Verification items for the finished model (mm, model axes). Face numbers are marked on the shaded views. A direction names the side the tool comes from. Coordinates: 2 decimals unless noted, no trailing zeros. Order: outer loops, then holes, each group sorted by start corner. A loop starts at its lowest first (then second) coordinate and runs counter-clockwise, first axis right, second up. Notation, with made-up numbers: (56, 34) - (111, 34) arc R31 ccw to (111, 59) - close; hole circle Ø3 at (43, -21.75). An arc over 180 degrees is marked (long way). Answer as CSV lines item,"result". Start each with the question number.
1. Set-up check for the marked faces 1, 2, 3 and 4: record each of +Z, -Z, +X, -X, +Y, -Y from which the full face is reachable in a straight line by a thin tool's end or side.
2. Section check C-C (z = -9.5). Record the cut outline in (x, y), and give its area (3 significant figures).
3. Material ranges on L1, parallel to X at y = -112.25, z = 10; L2, parallel to Y at x = 10, z = 9; L3, parallel to Y at x = 15.85, z = 10.5, recorded low to high. Write a range as [from, to].
4. Section check B-B (x = 37.5). Record the cut outline in (y, z).
5. Mould release check, pull along Y, two halves, no side actions. Record for the marked faces 5, 6, 7 and 8: pulls with the +Y half, pulls with the -Y half, needs draft (parallel to the pull), parting line crosses it, or undercut.
6. Go/stop test with flat-tipped pins: pin 1 (11 mm diameter, centred on x = 10, y = -10, fed in from -Z); pin 2 (6 mm diameter, centred on x = 26, z = -2.5, fed in from +Y); pin 3 (7.5 mm diameter, centred on y = -62, z = 3.5, fed in from +X). Record where each tip stops, or that it passes through.
7. Section check A-A (y = -10). Record the cut outline in (x, z), and give its area (3 significant figures).
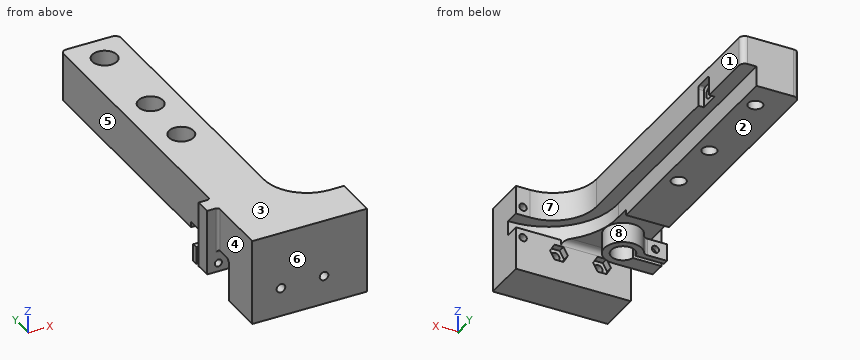
from build123d import *

# Parameters (mm, degrees)
BOSS_EXTRUDE1_DEPTH = 17
SKETCH3_W           = 40
SKETCH3_H           = 15
BOSS_EXTRUDE3_DEPTH = 13
FILLET1_R           = 15
SKETCH4_R           = 1.5000000000000004
SKETCH4_R_2         = 1.5000000000000007
CUT_EXTRUDE1_DEPTH  = 20
CUT_EXTRUDE2_DEPTH  = 2.5
SKETCH6_R           = 4.299999999999999
SKETCH6_R_2         = 4.299999999999998
SKETCH6_R_3         = 4.3
CUT_EXTRUDE3_DEPTH  = 12
SKETCH7_R           = 2.5000000000000004
SKETCH7_R_2         = 2.500000000000001
CUT_EXTRUDE4_DEPTH  = 12
CUT_EXTRUDE5_DEPTH  = 2
BOSS_EXTRUDE4_DEPTH = 23
BOSS_EXTRUDE5_DEPTH = 6
SKETCH11_W          = 6
SKETCH11_H          = 2
BOSS_EXTRUDE6_DEPTH = 4.419259302
SKETCH12_R          = 1.2500000000000002
CUT_EXTRUDE7_DEPTH  = 10
FILLET4_R           = 0.95
FILLET6_R           = 2
SKETCH13_R          = 6.500000000000007
SKETCH13_R_2        = 2.150000000000001
BOSS_EXTRUDE7_DEPTH = 1
SKETCH14_W          = 13.249650970727469
SKETCH14_H          = 1.5
CUT_EXTRUDE8_DEPTH  = 7
BOSS_EXTRUDE8_DEPTH = 10
SKETCH16_R          = 4.100000000000001
CUT_EXTRUDE9_DEPTH  = 6
CUT_EXTRUDE10_DEPTH = 5
SKETCH18_R          = 24.032057078793116
CUT_EXTRUDE11_DEPTH = 5
SKETCH20_R          = 1.3000000000000016
CUT_EXTRUDE12_DEPTH = 10
FILLET7_R           = 0.5
FILLET8_R           = 2
FILLET9_R           = 2
FILLET10_R          = 1
FILLET11_R          = 1
CUT_EXTRUDE15_DEPTH = 2
SKETCH24_R          = 2
CUT_EXTRUDE16_DEPTH = 5


with BuildPart() as part:
    # Sketch1 → Boss-Extrude1 (new body)
    with BuildSketch(Plane.XY):
        Polygon((0, 0), (1.531e-14, -125), (40.000000000000014, -125), (40.000000000000014, -110), (20.000000000000014, -110), (20.000000000000014, 0), align=None)
    extrude(amount=BOSS_EXTRUDE1_DEPTH)

    # Sketch3 → Boss-Extrude3 (add)
    with BuildSketch(Plane(origin=(0, 0, 0), x_dir=(-1, 0, 0), z_dir=(0, 0, -1))):
        with Locations((-20.000000000000014, -117.50000000000001)):
            Rectangle(SKETCH3_W, SKETCH3_H)
    extrude(amount=BOSS_EXTRUDE3_DEPTH)

    # Fillet1
    fillet1_edges = [part.edges().sort_by_distance(p)[0] for p in [
        (20.000000000000014, -110, 8.5),
    ]]
    fillet(fillet1_edges, radius=FILLET1_R)

    # Sketch4 → Cut-Extrude1 (cut)
    with BuildSketch(Plane.XZ.offset(125)):
        with Locations(Location((10.000000000000016, -2.999999999999999, 0), (0, 0, 270))):
            Circle(SKETCH4_R)
        with Locations(Location((25.000000000000014, -2.999999999999999, 0), (0, 0, 270))):
            Circle(SKETCH4_R_2)
    extrude(amount=-CUT_EXTRUDE1_DEPTH, mode=Mode.SUBTRACT)

    # Sketch5 → Cut-Extrude2 (cut)
    with BuildSketch(Plane(origin=(0, -110, 0), x_dir=(1, 0, 0), z_dir=(0, 1, 0))):
        Polygon((6.882308546376037, 3.0000000000000013), (8.441154273188026, 0.2999999999999986), (11.558845726812006, 0.2999999999999995), (13.117691453623996, 3.0000000000000018), (11.558845726812008, 5.7), (8.441154273188026, 5.699999999999998), align=None)
        Polygon((21.882308546376034, 2.999999999999999), (23.441154273188026, 0.2999999999999969), (26.558845726812, 0.29999999999999777), (28.117691453623994, 2.999999999999999), (26.558845726812, 5.6999999999999975), (23.441154273188022, 5.699999999999997), align=None)
    extrude(amount=-CUT_EXTRUDE2_DEPTH, mode=Mode.SUBTRACT)

    # Sketch6 → Cut-Extrude3 (cut)
    with BuildSketch(Plane.XY.offset(17)):
        with Locations((10.000000000000009, -10.000000000000002)):
            Circle(SKETCH6_R)
        with Locations((10.000000000000012, -40)):
            Circle(SKETCH6_R_2)
        with Locations((10.000000000000014, -60)):
            Circle(SKETCH6_R_3)
    extrude(amount=-CUT_EXTRUDE3_DEPTH, mode=Mode.SUBTRACT)

    # Sketch7 → Cut-Extrude4 (cut)
    with BuildSketch(Plane.XY.offset(5.000000000000001)):
        with Locations((10.000000000000009, -10.000000000000002)):
            Circle(SKETCH7_R)
        with Locations((10.000000000000012, -40)):
            Circle(SKETCH7_R_2)
        with Locations((10.000000000000014, -60)):
            Circle(SKETCH7_R_2)
    extrude(amount=-CUT_EXTRUDE4_DEPTH, mode=Mode.SUBTRACT)

    # Sketch8 → Cut-Extrude5 (cut)
    with BuildSketch(Plane(origin=(0, 0, 0), x_dir=(-1, 0, 0), z_dir=(0, 0, -1))):
        Polygon((-1.531e-14, -110), (-3.06e-15, -84.99999999999999), (-40.000000000000014, -84.99999999999999), (-40.000000000000014, -110), align=None)
    extrude(amount=-CUT_EXTRUDE5_DEPTH, mode=Mode.SUBTRACT)

    # Sketch9 → Boss-Extrude4 (add)
    with BuildSketch(Plane.XY.offset(17)):
        Polygon((-2.69e-15, -103.00000000000001), (-4, -103.00000000000001), (-4, -97.5), (0, -97.5), align=None)
    extrude(amount=-BOSS_EXTRUDE4_DEPTH)

    # Sketch10 → Boss-Extrude5 (add)
    with BuildSketch(Plane(origin=(0, 0, -5.999999999999998), x_dir=(-1, 0, 0), z_dir=(0, 0, -1))):
        with BuildLine():
            Line((4, -103.00000000000001), (-9.9, -103.00000000000001))
            ThreePointArc((-9.9, -103.00000000000001), (-15.308326913195994, -92.894448724536), (-3.8999999999999964, -94))
            Line((-3.8999999999999964, -94), (-0.41925930159213404, -94))
            Line((-0.41925930159213404, -94), (-0.41925930159213404, -96))
            Line((-0.41925930159213404, -96), (-5.931373033403113, -96))
            ThreePointArc((-5.931373033403113, -96), (-13.892119004323362, -96.24903017049799), (-6.025237793012059, -97.49308501111332))
            Line((-6.025237793012059, -97.49308501111332), (4, -97.5))
            Line((4, -97.5), (4, -103.00000000000001))
        make_face()
    extrude(amount=-BOSS_EXTRUDE5_DEPTH)

    # Sketch11 → Boss-Extrude6 (add)
    with BuildSketch(Plane.ZY.offset(-0.41925930159213404)):
        with Locations((-2.9999999999999982, -95)):
            Rectangle(SKETCH11_W, SKETCH11_H)
    extrude(amount=BOSS_EXTRUDE6_DEPTH)

    # Sketch12 → Cut-Extrude7 (cut)
    with BuildSketch(Plane(origin=(0, -94, 0), x_dir=(1, 0, 0), z_dir=(0, 1, 0))):
        with Locations((-0.05000000000000317, 2.9999999999999982)):
            Circle(SKETCH12_R)
    extrude(amount=-CUT_EXTRUDE7_DEPTH, mode=Mode.SUBTRACT)

    # Fillet4
    fillet4_edges = [part.edges().sort_by_distance(p)[0] for p in [
        (0, -97.5, 9.5),
        (-2.69e-15, -103.00000000000001, 9.5),
    ]]
    fillet(fillet4_edges, radius=FILLET4_R)

    # Fillet6
    fillet6_edges = [part.edges().sort_by_distance(p)[0] for p in [
        (20.000000000000014, 0, 8.5),
        (0, 0, 8.5),
    ]]
    fillet(fillet6_edges, radius=FILLET6_R)

    # Sketch13 → Boss-Extrude7 (add)
    with BuildSketch(Plane.XY):
        with Locations(Location((9.9, -96.5, 0), (0, 0, 175.588274214))):
            Circle(SKETCH13_R)
        with Locations((9.9, -96.5)):
            Circle(SKETCH13_R_2, mode=Mode.SUBTRACT)
    extrude(amount=BOSS_EXTRUDE7_DEPTH)

    # Sketch14 → Cut-Extrude8 (cut)
    with BuildSketch(Plane(origin=(0, 0, -5.999999999999998), x_dir=(-1, 0, 0), z_dir=(0, 0, -1))):
        with Locations((-2.6248254853637345, -96.75)):
            Rectangle(SKETCH14_W, SKETCH14_H)
    extrude(amount=-CUT_EXTRUDE8_DEPTH, mode=Mode.SUBTRACT)

    # Sketch15 → Boss-Extrude8 (add)
    with BuildSketch(Plane.XY):
        Polygon((0, -97.5), (2.5, -97.5), (2.5000000000000013, -103.00000000000001), (0, -103.00000000000001), align=None)
    extrude(amount=BOSS_EXTRUDE8_DEPTH)

    # Sketch16 → Cut-Extrude9 (cut)
    with BuildSketch(Plane(origin=(0, 0, -5.999999999999998), x_dir=(-1, 0, 0), z_dir=(0, 0, -1))):
        with Locations((-9.9, -96.5)):
            Circle(SKETCH16_R)
    extrude(amount=-CUT_EXTRUDE9_DEPTH, mode=Mode.SUBTRACT)

    # Sketch17 → Cut-Extrude10 (cut)
    with BuildSketch(Plane(origin=(20.000000000000014, 0, 0), x_dir=(0, 0, -1), z_dir=(1, 0, 0))):
        Polygon((0, 0), (-7, -8.6e-16), (-6.9999999999999885, -89.75912634068962), (0, -89.75912634068962), align=None)
    extrude(amount=-CUT_EXTRUDE10_DEPTH, mode=Mode.SUBTRACT)

    # Sketch18 → Cut-Extrude11 (cut)
    with BuildSketch(Plane(origin=(0, 0, 2), x_dir=(-1, 0, 0), z_dir=(0, 0, -1))):
        with Locations((-39.000000000000014, -91)):
            Circle(SKETCH18_R)
    extrude(amount=-CUT_EXTRUDE11_DEPTH, mode=Mode.SUBTRACT)

    # Sketch20 → Cut-Extrude12 (cut)
    with BuildSketch(Plane(origin=(0, -110, 0), x_dir=(1, 0, 0), z_dir=(0, 1, 0))):
        with Locations(Location((37.50000000000002, -9.999999999999998, 0), (0, 0, 270))):
            Circle(SKETCH20_R)
        with Locations(Location((37.50000000000002, 0.9999999999999974, 0), (0, 0, 90))):
            Circle(SKETCH20_R)
    extrude(amount=-CUT_EXTRUDE12_DEPTH, mode=Mode.SUBTRACT)

    # Fillet7
    fillet7_edges = [part.edges().sort_by_distance(p)[0] for p in [
        (2.500000000000001, -100.25, 2),
        (2.500000000000001, -100.25, 0),
    ]]
    fillet(fillet7_edges, radius=FILLET7_R)

    # Fillet8
    fillet8_edges = [part.edges().sort_by_distance(p)[0] for p in [
        (12.142354869960766, -110, 2),
    ]]
    fillet(fillet8_edges, radius=FILLET8_R)

    # Fillet9
    fillet9_edges = [part.edges().sort_by_distance(p)[0] for p in [
        (3.899999999999995, -94, -2.9999999999999982),
    ]]
    fillet(fillet9_edges, radius=FILLET9_R)

    # Fillet10
    fillet10_edges = [part.edges().sort_by_distance(p)[0] for p in [
        (1.025000000000007, -103.00000000000001, 2),
    ]]
    fillet(fillet10_edges, radius=FILLET10_R)

    # Fillet11
    fillet11_edges = [part.edges().sort_by_distance(p)[0] for p in [
        (1.0250000000000057, -97.5, 2),
    ]]
    fillet(fillet11_edges, radius=FILLET11_R)

    # Sketch23 → Cut-Extrude15 (cut)
    with BuildSketch(Plane(origin=(20.000000000000014, 0, 0), x_dir=(0, 0, -1), z_dir=(1, 0, 0))):
        with BuildLine():
            Line((-7, -21.5), (-7, -28.499999999999996))
            Line((-7, -28.499999999999996), (-12.999999999999993, -28.499999999999996))
            ThreePointArc((-12.999999999999993, -28.499999999999996), (-13.707106781186548, -28.207106781186543), (-14, -27.49999999999999))
            Line((-14, -27.49999999999999), (-14, -22.500000000000007))
            ThreePointArc((-14, -22.500000000000007), (-13.707106781186548, -21.79289321881345), (-12.999999999999993, -21.5))
            Line((-12.999999999999993, -21.5), (-7, -21.5))
        make_face()
    extrude(amount=-CUT_EXTRUDE15_DEPTH, mode=Mode.SUBTRACT)

    # Sketch24 → Cut-Extrude16 (cut)
    with BuildSketch(Plane(origin=(18.000000000000014, 0, 0), x_dir=(0, 0, -1), z_dir=(1, 0, 0))):
        with Locations((-10.5, -24.999999999999996)):
            Circle(SKETCH24_R)
    extrude(amount=-CUT_EXTRUDE16_DEPTH, mode=Mode.SUBTRACT)


solid = part.part
Evaluation:
1,face 1,"+Z, -Z, +X, +Y"
1,face 2,"-Z, +X, -X, +Y"
1,face 3,"+Z, +X, -X, +Y, -Y"
1,face 4,"+Z, -Z, -X, -Y"
2,outline,"(0, -125) - (40, -125) - (40, -110) - (0, -110) - close"
2,area,"600 mm²"
3,L1,"x = [0, 36.2], [38.8, 40]"
3,L2,"y = [-125, -64.3], [-55.7, -44.3], [-35.7, -14.3], [-5.7, 0]"
3,L3,"y = [-125, -27], [-23, 0]"
4,outline,"(-125, -13) - (-110, -13) - (-110, -2.3) - (-120, -2.3) - (-120, 0.3) - (-110, 0.3) - (-110, 2) - (-114.99, 2) - (-114.99, 7) - (-110, 7) - (-110, 8.7) - (-120, 8.7) - (-120, 11.3) - (-110, 11.3) - (-110, 17) - (-125, 17) - close"
5,face 5,"needs draft"
5,face 6,"pulls with the -Y half"
5,face 7,"pulls with the +Y half"
5,face 8,"undercut"
6,pin 1,"stops at z = 0"
6,pin 2,"stops at y = -110"
6,pin 3,"stops at x = 20"
7,outline,"(0, 0) - (7.5, 0) - (7.5, 5) - (5.7, 5) - (5.7, 17) - (0, 17) - close; (12.5, 0) - (15, 0) - (15, 7) - (20, 7) - (20, 17) - (14.3, 17) - (14.3, 5) - (12.5, 5) - close"
7,area,"177 mm²"
